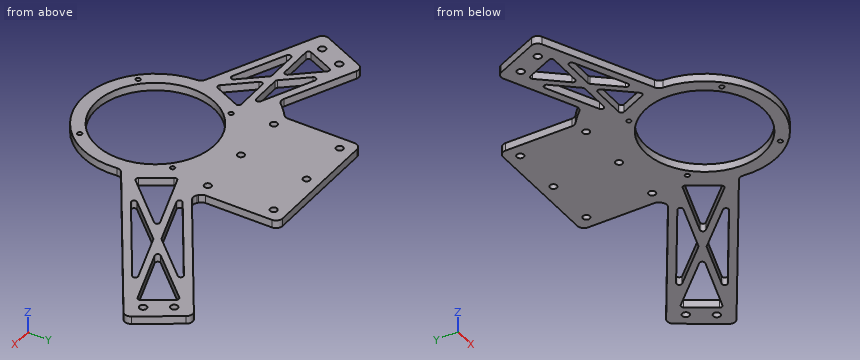
```python
from build123d import *

# Parameters (mm, degrees)
SKETCH8_R                      = 2.65
SKETCH8_R_2                    = 45
BOSS_EXTRUDE12_DEPTH           = 6
M5_CLEARANCE_HOLE3_D           = 5.5
M5_CLEARANCE_HOLE3_CSINK_D     = 5.55
M5_CLEARANCE_HOLE3_CSINK_ANGLE = 90
M3_CLEARANCE_HOLE2_D           = 3.4
M3_CLEARANCE_HOLE2_CSINK_D     = 3.45
M3_CLEARANCE_HOLE2_CSINK_ANGLE = 90
CUT_EXTRUDE12_DEPTH            = 234.420888215
FILLET16_R                     = 2
FILLET17_R                     = 2
FILLET13_R                     = 5


with BuildPart() as part:
    # Sketch8 → Boss-Extrude12 (new body)
    with BuildSketch(Plane.XY):
        with BuildLine():
            ThreePointArc((50, 66.988603427), (52.767551736, 64.83099932), (55.442106877, 62.559138214))
            Line((55.442106877, 62.559138214), (166.556546856, 133.975526494))
            Line((166.556546856, 133.975526494), (191.049389833, 95.86790727))
            Line((191.049389833, 95.86790727), (54.408449025, 8.044916078))
            ThreePointArc((54.408449025, 8.044916078), (3.903634668, -54.86129452), (-54.999385248, 0.260042998))
            Line((-54.999385248, 0.260042998), (-141.274934171, 39.741860486))
            Line((-141.274934171, 39.741860486), (-122.4246033, 80.933546856))
            Line((-122.4246033, 80.933546856), (-63.741426655, 54.07867895))
            ThreePointArc((-63.741426655, 54.07867895), (-57.235867879, 60.922314608), (-50, 66.988603427))
            Line((-50, 66.988603427), (-50, 125))
            Line((-50, 125), (50, 125))
            Line((50, 125), (50, 66.988603427))
        make_face()
        with Locations((-40, 65)):
            Circle(SKETCH8_R, mode=Mode.SUBTRACT)
        with Locations((0, 65)):
            Circle(SKETCH8_R, mode=Mode.SUBTRACT)
        with Locations((40, 65)):
            Circle(SKETCH8_R, mode=Mode.SUBTRACT)
        with Locations((0, 115)):
            Circle(SKETCH8_R, mode=Mode.SUBTRACT)
        with Locations((40, 115)):
            Circle(SKETCH8_R, mode=Mode.SUBTRACT)
        with Locations((-40, 115)):
            Circle(SKETCH8_R, mode=Mode.SUBTRACT)
        Circle(SKETCH8_R_2, mode=Mode.SUBTRACT)
    extrude(amount=BOSS_EXTRUDE12_DEPTH)

    # M5 Clearance Hole3 (through all)
    with Locations(Plane.XY.offset(6)):
        with Locations((-118.595460294, 65.269570227), (-126.91790218, 47.083395229), (164.983881766, 117.927186252), (175.797498975, 101.102630303)):
            CounterSinkHole(M5_CLEARANCE_HOLE3_D / 2, M5_CLEARANCE_HOLE3_CSINK_D / 2, counter_sink_angle=M5_CLEARANCE_HOLE3_CSINK_ANGLE)

    # M3 Clearance Hole2 (through all)
    with Locations(Plane.XY.offset(6)):
        with Locations((-35.355339059, 35.355339059), (35.355339059, 35.355339059), (35.355339059, -35.355339059), (-35.355339059, -35.355339059)):
            CounterSinkHole(M3_CLEARANCE_HOLE2_D / 2, M3_CLEARANCE_HOLE2_CSINK_D / 2, counter_sink_angle=M3_CLEARANCE_HOLE2_CSINK_ANGLE)

    # Sketch45 → Cut-Extrude12 (cut, through all)
    with BuildSketch(Plane.XY.offset(6)):
        Polygon((-116.995223223, 35.229285226), (-62.355834999, 10.224954562), (-83.893277645, 35.362478421), align=None)
        Polygon((-81.600914837, 40.371742739), (-103.138357483, 65.509266598), (-48.498969259, 40.504935934), align=None)
        Polygon((-55.848576336, 10.314784068), (-44.229729779, 35.522073712), (-77.331675357, 35.388880518), align=None)
        Polygon((-109.699959772, 65.482864501), (-88.162517126, 40.345340642), (-121.180939336, 40.212483522), align=None)
        Polygon((42.86381576, 44.280773431), (58.083519932, 20.600929819), (98.313351899, 63.188767486), align=None)
        Polygon((171.270720077, 93.349539589), (115.821183938, 74.441545533), (156.051015905, 117.0293832), align=None)
        Polygon((68.229920192, 24.060797821), (163.909288297, 85.556629544), (108.459752158, 66.648635488), align=None)
        Polygon((145.904615645, 113.569515198), (105.674783679, 70.981677531), (50.22524754, 52.073683476), align=None)
    extrude(amount=-CUT_EXTRUDE12_DEPTH, mode=Mode.SUBTRACT)

    # Fillet16
    fillet16_edges = [part.edges().sort_by_distance(p)[0] for p in [
        (-77.331675357, 35.388880518, 3),
        (-44.229729779, 35.522073712, 3),
        (-55.848576336, 10.314784068, 3),
        (-48.498969259, 40.504935934, 3),
        (-81.600914837, 40.371742739, 3),
        (-103.138357483, 65.509266598, 3),
        (-121.180939336, 40.212483522, 3),
        (-109.699959772, 65.482864501, 3),
        (-88.162517126, 40.345340642, 3),
        (-83.893277645, 35.362478421, 3),
        (-62.355834999, 10.224954562, 3),
        (-116.995223223, 35.229285226, 3),
    ]]
    fillet(fillet16_edges, radius=FILLET16_R)

    # Fillet17
    fillet17_edges = [part.edges().sort_by_distance(p)[0] for p in [
        (156.051015905, 117.0293832, 3),
        (171.270720077, 93.349539589, 3),
        (115.821183938, 74.441545533, 3),
        (108.459752158, 66.648635488, 3),
        (163.909288297, 85.556629544, 3),
        (68.229920192, 24.060797821, 3),
        (98.313351899, 63.188767486, 3),
        (58.083519932, 20.600929819, 3),
        (42.86381576, 44.280773431, 3),
        (50.22524754, 52.073683476, 3),
        (145.904615645, 113.569515198, 3),
        (105.674783679, 70.981677531, 3),
    ]]
    fillet(fillet17_edges, radius=FILLET17_R)

    # Fillet13
    fillet13_edges = [part.edges().sort_by_distance(p)[0] for p in [
        (55.442106877, 62.559138214, 3),
        (166.556546856, 133.975526494, 3),
        (191.049389833, 95.86790727, 3),
        (54.408449025, 8.044916078, 3),
        (-54.999385248, 0.260042998, 3),
        (-141.274934171, 39.741860486, 3),
        (-122.4246033, 80.933546856, 3),
        (-63.741426655, 54.07867895, 3),
        (-50, 66.988603427, 3),
        (-50, 125, 3),
        (50, 125, 3),
        (50, 66.988603427, 3),
    ]]
    fillet(fillet13_edges, radius=FILLET13_R)


solid = part.part
```
Model file for the job. Use its own axes, mm. Give positions to 0.01 mm unless a question says otherwise; leave off trailing zeros. Loops run counter-clockwise (first coordinate to the right, second up) from the corner with the lowest first, then second, coordinate; pieces in that order, holes last. Notation, with made-up numbers: (4, -31) -> (26, -31) arc R19 ccw to (26, -21) -> close; hole circle Ø7 at (82, 86.5). An arc over 180 degrees is marked (long way). Use CSV: the item, a comma, the result in double quotes. Start each with the question number.
1) Slice it at A-A on y = -7.5. Give the cut face in (x, z), plus the area to 3 significant figures.
2) Flat gauge pins, fed straight in: pin 1 Ø1.5 at (x, z) = (107, 3) entering from -Y; pin 2 Ø1 at (x, z) = (-83, 3.5) entering from +Y; pin 3 Ø1.8 at (y, z) = (83.5, 2) entering from +X. Where does each tip first touch, or does it go through?
3) Wall check: line 1 (Y direction, x = 0.5, z = 5.5); line 2 (Y direction, x = -102.5, z = 1); line 3 (X direction, y = 29, z = 2.25). Give the ranges that are in metal, low to high.
Computed values:
1,outline,"(-54.49, 0) -> (-44.37, 0) -> (-44.37, 6) -> (-54.49, 6) -> close; (44.37, 0) -> (54.49, 0) -> (54.49, 6) -> (44.37, 6) -> close"
1,area,"121 mm^2"
2,pin 1,"stops at y = 41.36"
2,pin 2,"stops at y = 63.12"
2,pin 3,"stops at x = 173.21"
3,line 1,"y = -55 to -45, 45 to 62.4, 67.6 to 112.4, 117.6 to 125"
3,line 2,"y = 22 to 28.6, 35.29 to 40.29, 57.08 to 71.82"
3,line 3,"x = -117.8 to -103.38, -78.44 to -71.86, -47.24 to -34.41, 34.41 to 52.69, 66.02 to 87.01"
